Input: dimensioned drawing with shaded views. Units: mm. Origin: part minimum x, y, z. Round coordinates to 2 decimals unless told otherwise and drop trailing zeros. Loops run counter-clockwise (first coordinate to the right, second up) from the corner with the lowest first, then second, coordinate; pieces in that order, holes last. Notation, with made-up numbers: (-27, 27.5) - (-3, 27.5) arc R29 cw to (-3, 64.5) - close; hole circle Ø2 at (-29, 28.5). An arc over 180 degrees is marked (long way). One line per question, with ' | ' between items.
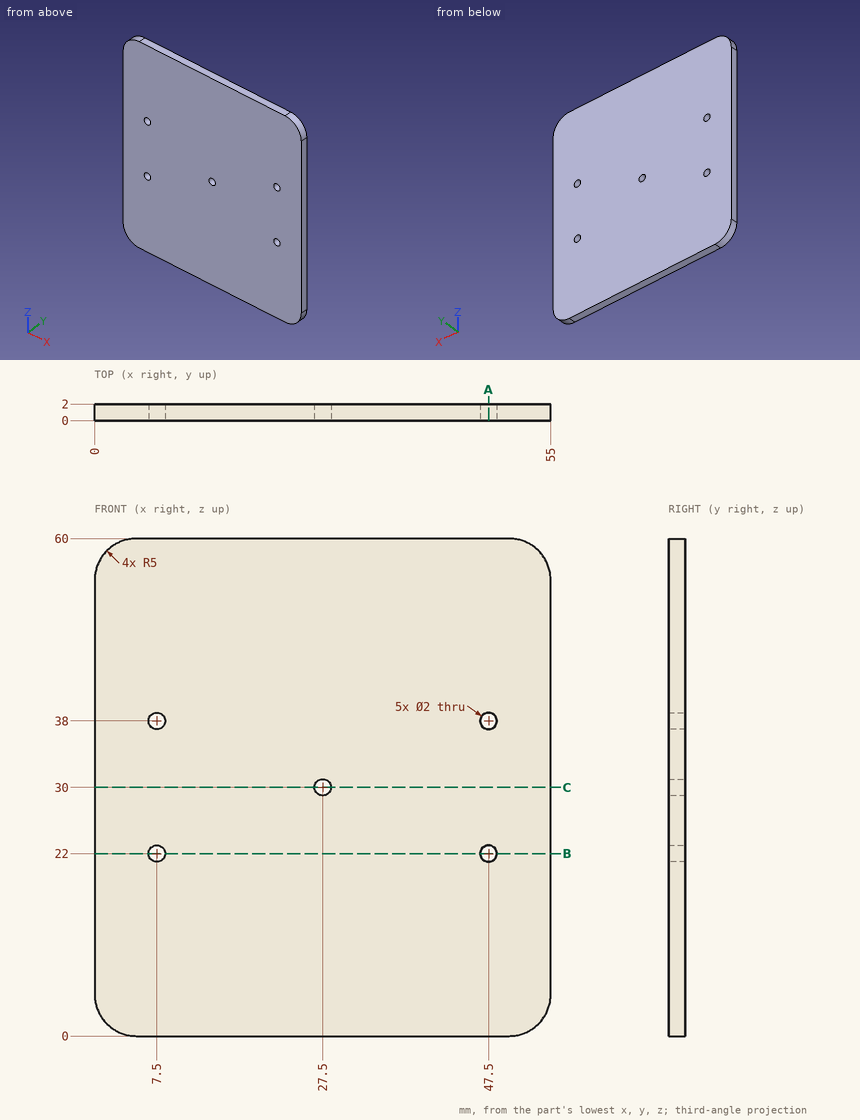
1. Material intervals for probe 1 along X at (y, z) = (1.5, 38); probe 2 along Z at (x, y) = (47.5, 1.4); probe 3 along X at (y, z) = (0.95, 30), sorted ascending.
Worked out:
probe 1: x = 0 to 6.5, 8.5 to 46.5, 48.5 to 55 | probe 2: z = 0 to 21, 23 to 37, 39 to 60 | probe 3: x = 0 to 26.5, 28.5 to 55
2. Contact query for flat-ended pins moving along their axis: P1, Ø1.2, axis at x = 27.5, z = 30, coming from the -Y side; P2, Ø3, axis at x = 19, z = 25.5, coming from the -Y side. Output: stop coordinate, or through.
Worked out:
P1: passes through | P2: stops at y = 0
3. Section query B-B, the plane z = 22. Return loops of the section in (x, y).
Worked out:
outline: (0, 0) - (6.5, 0) - (6.5, 2) - (0, 2) - close; (8.5, 0) - (46.5, 0) - (46.5, 2) - (8.5, 2) - close; (48.5, 0) - (55, 0) - (55, 2) - (48.5, 2) - close
4. Section query A-A, the plane x = 47.5. Return loops of the section in (y, z).
Worked out:
outline: (0, 0) - (2, 0) - (2, 21) - (0, 21) - close; (0, 23) - (2, 23) - (2, 37) - (0, 37) - close; (0, 39) - (2, 39) - (2, 60) - (0, 60) - close
5. Section query C-C, the plane z = 30. Return loops of the section in (x, y), plus the area to 3 significant figures.
Worked out:
outline: (0, 0) - (26.5, 0) - (26.5, 2) - (0, 2) - close; (28.5, 0) - (55, 0) - (55, 2) - (28.5, 2) - close | area: 106 mm2
